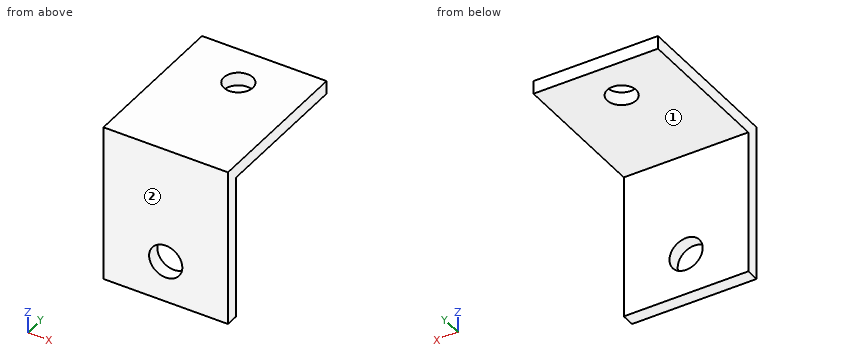
from build123d import *

# Parameters (mm, degrees)
SKETCH1_W               = 30
SKETCH1_H               = 38
BOSS_EXTRUDE1_DEPTH     = 3.175
SKETCH2_W               = 30
SKETCH2_H               = 3.175
BOSS_EXTRUDE2_DEPTH     = 34.825
SKETCH3_R               = 4
CUT_EXTRUDE1_DEPTH      = 60.638751035
SKETCH4_R               = 4
CUT_EXTRUDE2_DEPTH      = 58.667679423
CROQUIS4_R              = 4
CROQUIS4_R_2            = 3.5
SALIENTE_EXTRUIR2_DEPTH = 5
CROQUIS5_W              = 3.979032683
CROQUIS5_H              = 10.100326852
CORTAR_EXTRUIR1_DEPTH   = 36


with BuildPart() as part:
    # Sketch1 → Boss-Extrude1 (new body)
    with BuildSketch(Plane.XY):
        with Locations((15, 19)):
            Rectangle(SKETCH1_W, SKETCH1_H)
    extrude(amount=BOSS_EXTRUDE1_DEPTH)

    # Sketch2 → Boss-Extrude2 (add)
    with BuildSketch(Plane(origin=(0, 0, 0), x_dir=(-1, 0, 0), z_dir=(0, 0, -1))):
        with Locations((-15, 1.5875)):
            Rectangle(SKETCH2_W, SKETCH2_H)
    extrude(amount=BOSS_EXTRUDE2_DEPTH)

    # Sketch3 → Cut-Extrude1 (cut, through all)
    with BuildSketch(Plane(origin=(0, 0, 0), x_dir=(-1, 0, 0), z_dir=(0, 0, -1))):
        with Locations((-15, 28)):
            Circle(SKETCH3_R)
    extrude(amount=-CUT_EXTRUDE1_DEPTH, mode=Mode.SUBTRACT)

    # Sketch4 → Cut-Extrude2 (cut, through all)
    with BuildSketch(Plane(origin=(0, 3.175, 0), x_dir=(1, 0, 0), z_dir=(0, 1, 0))):
        with Locations(Location((15, 24.825, 0), (0, 0, 180))):
            Circle(SKETCH4_R)
    extrude(amount=-CUT_EXTRUDE2_DEPTH, mode=Mode.SUBTRACT)

    # Croquis4 → Saliente-Extruir2 (add)
    with BuildSketch(Plane(origin=(0, 0, 0), x_dir=(-1, 0, 0), z_dir=(0, 0, -1))):
        with Locations((-15, 28)):
            Circle(CROQUIS4_R)
        with Locations((-15, 28)):
            Circle(CROQUIS4_R_2, mode=Mode.SUBTRACT)
    extrude(amount=-SALIENTE_EXTRUIR2_DEPTH)

    # Croquis5 → Cortar-Extruir1 (cut)
    with BuildSketch(Plane.ZY):
        with Locations((5.164516342, 27.585777405)):
            Rectangle(CROQUIS5_W, CROQUIS5_H)
    extrude(amount=-CORTAR_EXTRUIR1_DEPTH, mode=Mode.SUBTRACT)


solid = part.part
Can you work these out from the model? Positions are in its coordinate system, mm. Face numbers are marked on the shaded views. A direction names the side the tool comes from. Give positions to 0.01 mm unless a question says otherwise; leave off trailing zeros. Order: outer loops, then holes, each group sorted by start corner. A loop starts at its lowest first (then second) coordinate and runs counter-clockwise, first axis right, second up. Notation, with made-up numbers: (1.25, 21.25) - (27.25, 21.25) arc R18 ccw to (27.25, 25.25) - close; hole circle Ø11 at (-6.75, 73.25). An arc over 180 degrees is marked (long way). Write each question's results on one line, items separated by ' | '.
1) Please list where these lines run through material, in increasing order: line 1 along Z through (x, y) = (15, 2.35) (3 decimals); line 2 along Y through (x, z) = (3.25, -14) (3 decimals). Write a range as [from, to].
Final values:
line 1: z = [-34.825, -28.825], [-20.825, 3.175] | line 2: y = [0, 3.175]
2) Suppose I cut it at A-A, the plane x = 15. Write out the boundary of the cut face in (y, z) (3 decimals), then the cut area to 3 significant figures.
Final values:
outline: (0, -34.825) - (3.175, -34.825) - (3.175, -28.825) - (0, -28.825) - close; (0, -20.825) - (3.175, -20.825) - (3.175, 0) - (24.5, 0) - (24.5, 3.175) - (0, 3.175) - close; (31.5, 0) - (38, 0) - (38, 3.175) - (31.5, 3.175) - close | area: 184 mm^2
3) Suppose I cut it at D-D, the plane z = -30. Write out the boundary of the cut face in (x, y) (3 decimals).
Final values:
outline: (0, 0) - (30, 0) - (30, 3.175) - (0, 3.175) - close
4) Suppose I cut it at C-C, the plane x = 27.25. Write out the boundary of the cut face in (y, z) (3 decimals).
Final values:
outline: (0, -34.825) - (3.175, -34.825) - (3.175, 0) - (38, 0) - (38, 3.175) - (0, 3.175) - close
5) Suppose I cut it at B-B, the plane y = 28. Write out the boundary of the cut face in (x, z) (3 decimals).
Final values:
outline: (0, 0) - (11.5, 0) - (11.5, 3.175) - (0, 3.175) - close; (18.5, 0) - (30, 0) - (30, 3.175) - (18.5, 3.175) - close
6) On a 3-axis mill with a long thin cutter (end or side, diameter ignored), from which of +Z, -Z, +X, -X, +Y, -Y can I reach the whole of each face in a straight line? I mean the marked faces 1 and 2. Say none if no direction works.
Final values:
face 1: -Z, +X, -X, +Y | face 2: +Z, -Z, +X, -X, -Y
7) I'm going to push flat-ended pins straight in: pin 1 Ø8 at (x, z) = (4.5, -7.5) entering from +Y (3 decimals); pin 2 Ø4 at (x, y) = (15, 28) entering from -Z; pin 3 Ø3 at (x, y) = (3.5, 8.5) entering from -Z. Where does each tip first touch, or does it pass through?
Final values:
pin 1: stops at y = 3.175 | pin 2: passes through | pin 3: stops at z = 0
